Design review of the part built by this model. Coordinates are the model's own, in mm. A direction names the side the tool comes from. Coordinates: 2 decimals unless noted, no trailing zeros. Write each loop counter-clockwise with the first axis right and the second up, starting at its lowest first coordinate (ties: lowest second). Pieces come first, ordered by that corner, then holes. Notation, with made-up numbers: (57.25, 70) -> (89.25, 70) arc R29 ccw to (89.25, 108) -> close; hole circle Ø1 at (6, -31). An arc over 180 degrees is marked (long way). One line per question, with ' | ' between items. Start each with the question number.
Q1. Wall thickness on probe 1 along X at (y, z) = (25.5, 66); probe 2 along Z at (x, y) = (12.5, 3): over which ranges is each line inside the solid? List them lowest first.
Q2. For P1, Ø14, axis at y = -34, z = 53, coming from the -X side; P2, Ø1, axis at x = 40, z = 72.5, coming from the +Y side; P3, Ø14, axis at x = -33.5, z = 52.5, coming from the -Y side, all flat-tipped, find the tip position at first contact; note any pin that passes through.
Q3. Add section C-C on y = -31. State the section outline as (x, z) points, and give its area (3 significant figures).
Q4. Add section B-B on x = 2.5. State the section outline as (y, z) points, and give its area (3 significant figures).
Q5. Add section A-A on z = 74.5. State the section outline as (x, y) points, and give its area (3 significant figures).
Q6. For faces 1 (the flat face through (-1, 3, 0)), 2 (the flat face through (0, 28, 46)), 3 (the flat face through (0, -24, 46)), 4 (the flat face through (5, -23, 46)), 5 (the flat face through (28, 5, 46)), list the 3-axis set-ups (+Z, -Z, +X, -X, +Y, -Y) from which the entire face can be reached by the end or side of a thin tool; tool diameter is ignored.
from build123d import *

# Parameters (mm, degrees)
P_IDAT_VYSUNUT_M1_DEPTH = 93.2
SKICA2_R                = 2.5
P_IDAT_VYSUNUT_M2_DEPTH = 70


with BuildPart() as part:
    # Skica1 → Přidat vysunutím1 (new body)
    with BuildSketch(Plane.XY):
        Polygon((0, 0), (-46.5, 0), (-46.5, 5), (0, 5), (0, 51.5), (5, 51.5), (5, 5), (51.5, 5), (51.5, 0), (5, 0), (5, -46.5), (0, -46.5), align=None)
    extrude(amount=P_IDAT_VYSUNUT_M1_DEPTH)

    # Skica2 → Přidat vysunutím2 (add)
    with BuildSketch(Plane.XY):
        with Locations((2.5, 2.536963061)):
            Circle(SKICA2_R)
    extrude(amount=-P_IDAT_VYSUNUT_M2_DEPTH)


solid = part.part
Output values:
1) probe 1: x = 0 to 5 | probe 2: z = 0 to 93.2
2) P1: stops at x = 0 | P2: stops at y = 5 | P3: stops at y = 0
3) outline: (0, 0) -> (5, 0) -> (5, 93.2) -> (0, 93.2) -> close | area: 466 mm2
4) outline: (-46.5, 0) -> (0.04, 0) -> (0.04, -70) -> (5.04, -70) -> (5.04, 0) -> (51.5, 0) -> (51.5, 93.2) -> (-46.5, 93.2) -> close | area: 9,480 mm2
5) outline: (-46.5, 0) -> (0, 0) -> (0, -46.5) -> (5, -46.5) -> (5, 0) -> (51.5, 0) -> (51.5, 5) -> (5, 5) -> (5, 51.5) -> (0, 51.5) -> (0, 5) -> (-46.5, 5) -> close | area: 955 mm2
6) face 1: -Z | face 2: +Z, -Z, -X, +Y | face 3: +Z, -Z, -X, -Y | face 4: +Z, -Z, +X, -Y | face 5: +Z, -Z, +X, +Y
